```python
from build123d import *

# Parameters (mm, degrees)
BOSS_EXTRUDE1_DEPTH = 2


with BuildPart() as part:
    # Sketch1 → Boss-Extrude1 (new body)
    with BuildSketch(Plane(origin=(0, 0, 0), x_dir=(1, 0, 0), z_dir=(0, 1, 0))):
        with BuildLine():
            Line((24, 0), (48, 0))
            add(Edge.make_bspline(
                [(48, 0), (89.099365724, 0.874773385), (86.374059044, -51.603142983), (121.547837425, -58.986384407)],
                knots=[0, 0, 0, 0, 1, 1, 1, 1], degree=3))
            Line((121.547837425, -58.986384407), (221.547837425, -58.986384407))
            Line((221.547837425, -58.986384407), (221.547837425, -51.986384407))
            Line((221.547837425, -51.986384407), (122.313023704, -51.986384407))
            add(Edge.make_bspline(
                [(71.125998731, 1.232568174), (72.898809563, 0.181682333), (76.459813959, -2.315666191), (81.189700312, -6.726275017), (86.891376041, -13.416403627), (92.807836153, -22.347568969), (98.129903366, -31.060917059), (102.469737091, -37.345221684), (105.842818581, -41.580534372), (109.401004038, -45.224982649), (112.577237242, -47.710854013), (115.306225207, -49.358382328), (117.470523961, -50.422439309), (119.399803514, -51.164246751), (121.027397151, -51.664895321), (121.885844483, -51.886407758), (122.313023704, -51.986384407)],
                knots=[0.193856357, 0.193856357, 0.193856357, 0.193856357, 0.248016758, 0.310020948, 0.372025138, 0.496033517, 0.620041896, 0.682046086, 0.744050275, 0.806054465, 0.868058655, 0.899060749, 0.930062844, 0.961064939, 0.976565986, 0.992067034, 0.992067034, 0.992067034, 0.992067034], degree=3))
            add(Edge.make_bspline(
                [(48.443659708, 40.664433584), (50.620366821, 24.429534749), (58.981751845, 11.448277847), (71.125998731, 1.232568174)],
                knots=[0.080375853, 0.080375853, 0.080375853, 0.080375853, 1, 1, 1, 1], degree=3))
            ThreePointArc((48.443659708, 40.664433584), (46.780254452, 43.763121571), (43.488003544, 45))
            Line((43.488003544, 45), (24, 45))
            Line((24, 45), (24, 0))
        make_face()
    boss_extrude1 = extrude(amount=BOSS_EXTRUDE1_DEPTH)

    # Mirror1: Boss-Extrude1 across plane
    add(boss_extrude1.mirror(Plane(origin=(24, 2, -45), x_dir=(0, 0, 1), z_dir=(1, 0, 0))))


solid = part.part
```
Work out the finished part from the listing and answer in its coordinate system (mm). Give positions to 0.01 mm unless a question says otherwise; leave off trailing zeros. Loops run counter-clockwise (first coordinate to the right, second up) from the corner with the lowest first, then second, coordinate; pieces in that order, holes last. Notation, with made-up numbers: (88.25, 73.5) - (135.25, 73.5) arc R30 ccw to (135.25, 102.5) - close; hole circle Ø3 at (8.5, 40). An arc over 180 degrees is marked (long way). One line per question, with ' | ' between items.
(1) Straight lines are drawn through the part: probe 1 along Z at (x, y) = (204, 1.1); probe 2 along X at (y, z) = (1.8, 39); probe 3 along X at (y, z) = (0.25, 18). For each, find the intervals that lie inside material, in ascending order.
Recorded:
probe 1: z = 51.99 to 58.99 | probe 2: x = -55.81 to -47.12, 95.12 to 103.81 | probe 3: x = -41.88 to -33.32, 81.32 to 89.88
(2) Each of these flat-tipped pins is pushed along its axis until it touches: pin 1 Ø1 at (x, y) = (-122.5, 1) entering from -Z; pin 2 Ø0.6 at (x, y) = (13.5, 1) entering from +Z. Where does it stop, or does it pass through?
Recorded:
pin 1: stops at z = 51.99 | pin 2: stops at z = 0
(3) The part is cut by section A-A (x = -85). Write down the section's boundary in (y, z), then the cut area to 3 significant figures.
Recorded:
outline: (0, 51.99) - (2, 51.99) - (2, 58.99) - (0, 58.99) - close | area: 14.0 mm²
